Source: CAD feature listing. Evaluate the final solid. Frame: model axes, mm. Face numbers are marked on the shaded views. Coordinates: 2 decimals unless noted, no trailing zeros. Write each loop counter-clockwise with the first axis right and the second up, starting at its lowest first coordinate (ties: lowest second). Pieces come first, ordered by that corner, then holes. Notation, with made-up numbers: (-35, 55.25) - (20, 55.25) arc R6 ccw to (20, 61.25) - close; hole circle Ø10 at (38.25, 67.25). An arc over 180 degrees is marked (long way). One line per item, written item: value.
Solid Edge part; units mm, degrees
sketch "Sketch1" plane through (0, 0, 0) normal (0, -1, 0) x (1, 0, 0)
  line L0 (63, -0.6391) -> (70.8743, -5.9205)
  arc A0 (70.8743, -5.9205) -> (75.5003, -6.7985) centre (74.2164, -0.9375) ccw
  line L1 (75.5003, -6.7985) -> (77.1662, -6.4336)
  arc A1 (77.1662, -6.4336) -> (78.3755, -10.8236) centre (77.654, -8.6608) cw
  line L2 (68.7638, -13.9467) -> (78.3755, -10.8236)
  arc A2 (63.7302, -13.3286) -> (68.7638, -13.9467) centre (66.9097, -8.2403) ccw
  line L3 (61.6545, -12.0316) -> (63.7302, -13.3286)
  arc A3 (58.2681, -11.1234) -> (61.6545, -12.0316) centre (58.4749, -17.1199) cw
  line L4 (36.7927, -11.8642) -> (58.2681, -11.1234)
  arc A4 (36.7927, -11.8642) -> (35.352, -10.0047) centre (36.7427, -10.4151) cw
  line L5 (35.352, -10.0047) -> (36.3854, -6.5024)
  arc A5 (34.9947, -4.642) -> (36.3854, -6.5024) centre (34.9947, -6.092) cw
  line L6 (6.1997, -4.642) -> (34.9947, -4.642)
  line L7 (-0.8003, -3.026) -> (6.1997, -4.642)
  arc A6 (0, 3.13) -> (-0.8003, -3.026) centre (0, 0) ccw
  line L8 (0, 3.13) -> (31.1, 3.13)
  line L9 (31.1, 3.13) -> (46.5, 1.7827)
  line L10 (46.5, 1.7827) -> (63, -0.6391)
  circle A7 centre (44.1, -5.6) radius 0.95
  circle A8 centre (39.75, -8.75) radius 0.95
  circle A9 centre (77.1662, -8.7136) radius 0.95
  circle A10 centre (0, 0) radius 0.95
extrude "Protrusion1" add sketch "Sketch1" along normal mid plane 36
fillet "Round_1" radius 2 4 edges at (31.1, 0, 3.13) (46.5, 0, 1.7827) (63, 0, -0.6391) (6.1997, 0, -4.642)
sketch "Sketch2" plane through (15.5063, 0, 3.13) normal (0, 0, 1) x (-1, 0, 0)
  line L0 (25.1795, 16) -> (-74.8205, 16)
  line L1 (-74.8205, 16) -> (-74.8205, -16)
  line L2 (-74.8205, -16) -> (25.1795, -16)
  line L3 (25.1795, -16) -> (25.1795, 16)
extrude "Cutout1" cut sketch "Sketch2" against normal through all
sketch "Sketch3" plane through (38.402, -18, -5.5552) normal (0, -1, 0) x (1, 0, 0)
  circle A0 centre (20.248, -0.1948) radius 3.75
extrude "Protrusion2" add sketch "Sketch3" against normal up to surface (32 mm away) from surface at -2
properties material "Stainless Steel, 420"
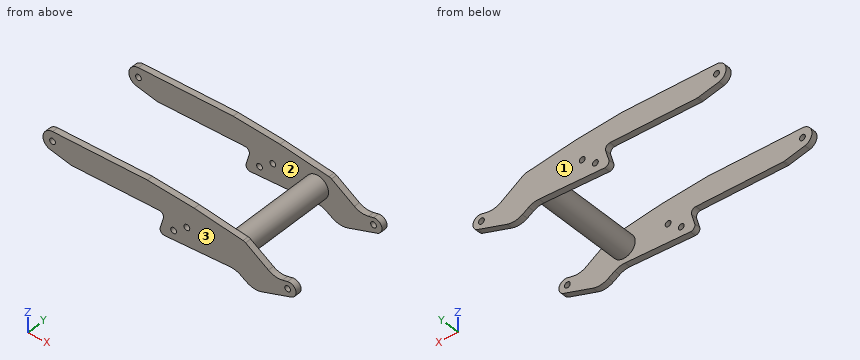
1) Section query A-A on x = 17.5. Output: boundary loops of the cut face in (y, z), then the cut area to 3 significant figures.
Values found:
outline: (-18, -4.64) - (-16, -4.64) - (-16, 3.13) - (-18, 3.13) - close; (16, -4.64) - (18, -4.64) - (18, 3.13) - (16, 3.13) - close
area: 31.1 mm2
2) Material intervals for line 1 (Y direction, x = 17, z = 2); line 2 (X direction, y = 17.15, z = -8.75); line 3 (X direction, y = -6.5, z = -6), sorted ascending.
Values found:
line 1: -18 to -16, 16 to 18
line 2: 35.72 to 38.8, 40.7 to 76.22, 78.12 to 79.93
line 3: 54.91 to 62.39
3) Section query B-B on x = 39.75. Output: boundary loops of the cut face in (y, z).
Values found:
outline: (-18, -11.76) - (-16, -11.76) - (-16, -9.7) - (-18, -9.7) - close; (-18, -7.8) - (-16, -7.8) - (-16, 2.37) - (-18, 2.37) - close; (16, -11.76) - (18, -11.76) - (18, -9.7) - (16, -9.7) - close; (16, -7.8) - (18, -7.8) - (18, 2.37) - (16, 2.37) - close
4) Contact query for flat-ended pins moving along their axis: P1, Ø2, axis at x = 20, y = 17, coming from the -Z side; P2, Ø6, axis at y = -9.5, z = -8.5, coming from the +X side; P3, Ø6, axis at y = -14, z = -12, coming from the -X side. Output: stop coordinate, or through.
Values found:
P1: z = -4.64
P2: x = 62.4
P3: x = 35.29
5) Section query D-D on x = 67.5. Output: boundary loops of the cut face in (y, z), then the cut area to 3 significant figures.
Values found:
outline: (-18, -14.21) - (-16, -14.21) - (-16, -3.66) - (-18, -3.66) - close; (16, -14.21) - (18, -14.21) - (18, -3.66) - (16, -3.66) - close
area: 42.2 mm2
6) Draft query along Y for the marked faces 1, 2 and 3. Return one class per face: released by +Y, released by -Y, zero draft, split by the parting line, or undercut.
Values found:
face 1: released by +Y
face 2: undercut
face 3: released by -Y
7) Section query C-C on y = 9. Output: boundary loops of the cut face in (x, z), then the cut area to 3 significant figures.
Values found:
outline: circle Ø7.5 at (58.65, -5.75)
area: 44.2 mm2
